CAD build for the part. Positions are in the model's coordinates, mm. Coordinates: 2 decimals unless noted, no trailing zeros. Order: outer loops, then holes, each group sorted by start corner. A loop starts at its lowest first (then second) coordinate and runs counter-clockwise, first axis right, second up. Notation, with made-up numbers: (45.5, 89.25) - (97.5, 89.25) arc R26 ccw to (97.5, 116.25) - close; hole circle Ø10 at (13.5, -22.5). An arc over 180 degrees is marked (long way). Return JSON: item names as keys, results as strings.
Autodesk Inventor part; units mm, degrees
ref_plane "YZ Plane" through (0, 0, 0) normal (1, 0, 0) x (0, 1, 0)
ref_plane "XZ Plane" through (0, 0, 0) normal (0, 1, 0) x (-1, 0, 0)
ref_plane "XY Plane" through (0, 0, 0) normal (0, 0, 1) x (1, 0, 0)
sketch "Sketch1" plane through (0, 0, 0) normal (0, 1, 0) x (-1, 0, 0)
  line L0 (-50.8, -26.6065) -> (50.8, -26.6065)
  line L1 (50.8, -26.6065) -> (50.8, 26.6065)
  line L2 (50.8, 26.6065) -> (-50.8, 26.6065)
  line L3 (-50.8, 26.6065) -> (-50.8, -26.6065)
  line L4 (-50.8, -26.6065) -> (50.8, 26.6065) construction
  line L5 (50.8, -26.6065) -> (-50.8, 26.6065) construction
  point P0 (0, 0)
  dimension "d0" = 101.6
  dimension "d1" = 53.213
extrude "Extrusion1" add sketch "Sketch1" along normal blind 1.651
sketch "Sketch3" plane through (0, 1.651, 0) normal (0, 1, 0) x (1, 0, 0)
  line L0 (50.8, 26.6065) -> (-50.8, 26.6065)
  line L1 (-50.8, 26.6065) -> (-50.8, -26.6065)
  circle A0 centre (-36.83, 24.0665) radius 1.5875
  circle A1 centre (45.72, 24.0665) radius 1.5875
  circle A2 centre (-35.56, -24.1935) radius 1.5875
  circle A3 centre (39.37, -24.1935) radius 1.5875
  point P0 (0, 0)
  dimension "d4" = 3.175
  dimension "d5" = 2.54
  dimension "d6" = 13.97
  dimension "d7" = 3.175
  dimension "d10" = 3.175
  dimension "d12" = 3.175
  dimension "d35" = 50.8
  dimension "d36" = 15.24
  dimension "d37" = 2.54
  dimension "d38" = 96.52
  dimension "d39" = 50.8
  dimension "d40" = 90.17
extrude "Extrusion2" cut sketch "Sketch3" against normal blind 1.651
chamfer "Chamfer1" distance 3.175 angle 45 1 edges at (50.8, 0.8255, -26.6065) measured on face at (16.9333, 0.5503, -26.6065)
sketch "Sketch5" plane through (0, 1.651, 0) normal (0, 1, 0) x (1, 0, 0)
  line L0 (-50.8, 26.6065) -> (50.6857, 26.8236) construction
  line L1 (50.6857, 26.8236) -> (50.8, -26.6065) construction
  line L2 (50.8, -26.6065) -> (-50.6857, -26.8236) construction
  line L3 (-50.6857, -26.8236) -> (-50.8, 26.6065) construction
  point P0 (0, 0)
decal "Decal1"
sketch "Sketch6" plane through (0, 1.651, 0) normal (0, 1, 0) x (1, 0, 0)
  line L0 (47.625, 26.6065) -> (50.8, 23.4315)
  line L1 (-50.8, -26.6065) -> (50.8, -26.6065)
  line L2 (50.8, -26.6065) -> (50.8, 23.4315)
  line L3 (50.8, -11.6321) -> (48.5549, -13.8772)
  line L4 (48.5549, -13.8772) -> (48.5549, -26.6065)
  point P0 (0, 0)
extrude "Extrusion3" cut sketch "Sketch6" against normal blind 1.651
chamfer "Chamfer2" distance 2.286 angle 45 1 edges at (48.5549, 0.8255, 26.6065)
sketch "Sketch7" plane through (0, 0, 0) normal (0, -1, 0) x (1, 0, 0)
  line L0 (-50.8, 26.6065) -> (50.7588, 26.6844) construction
  line L1 (50.7588, 26.6844) -> (50.8, -27.0821) construction
  line L2 (50.8, -27.0821) -> (-50.7588, -27.1599) construction
  line L3 (-50.7588, -27.1599) -> (-50.8, 26.6065) construction
  point P0 (0, 0)
decal "Decal2"
properties part number "PCB-FIXED"
Item 1: Mould opens along Z. For faces 1 (the cylindrical face through (-35.977, 0.837, -25.405)), 2 (the flat face through (49.19, 0.84, -25.04)), 3 (the cylindrical face through (-34.827, 0.837, 25.602)), 4 (the flat face through (47.396, 0.814, 25.48)) say: released by +Z, released by -Z, zero draft, split by the parting line, or undercut.
Findings below:
{"face 1": "undercut", "face 2": "released by -Z", "face 3": "undercut", "face 4": "released by +Z"}
Item 2: Wall check: L1, parallel to Z at x = -35.56, y = 0.4; L2, parallel to Z at x = 39.37, y = 0.55; L3, parallel to X at y = 0.2, z = 23. Give the ranges that are in metal, low to high. Write a range as [from, to].
Findings below:
{"L1": "z = [-26.61, -25.02], [-23.11, 22.61], [25.78, 26.61]", "L2": "z = [-26.61, 22.61], [25.78, 26.61]", "L3": "x = [-50.8, -36.61], [-34.51, 38.32], [40.42, 48.55]"}
Item 3: Drop a flat-ended pin along its axis: P1, Ø2.5, axis at x = 45.72, z = -24.07, coming from the -Y side. Give the stop position or say it passes through.
Findings below:
{"P1": "passes through"}
Item 4: Band-saw the part on B-B, the plane z = 15. List the corners of the cut face in (x, y).
Findings below:
{"outline": "(-50.8, 0) - (48.55, 0) - (48.55, 1.65) - (-50.8, 1.65) - close"}
Item 5: Band-saw the part on A-A, the plane x = 39.37. List the corners of the cut face in (y, z), then the cut area to 3 significant figures.
Findings below:
{"outline": "(0, -26.61) - (1.65, -26.61) - (1.65, 22.61) - (0, 22.61) - close; (0, 25.78) - (1.65, 25.78) - (1.65, 26.61) - (0, 26.61) - close", "area": "82.6 mm²"}
